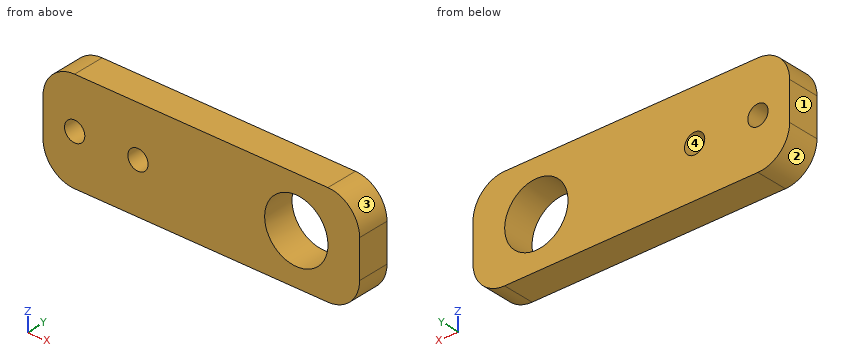
from build123d import *

# Parameters (mm, degrees)
SKETCH1_W           = 50
SKETCH1_H           = 16
SKETCH1_R           = 5
SKETCH1_R_2         = 1.6
BOSS_EXTRUDE1_DEPTH = 5
FILLET1_R           = 5


with BuildPart() as part:
    # Sketch1 → Boss-Extrude1 (new body)
    with BuildSketch(Plane(origin=(0, 0, 0), x_dir=(1, 0, 0), z_dir=(0, 1, 0))):
        with Locations((25, 8)):
            Rectangle(SKETCH1_W, SKETCH1_H)
        with Locations(Location((40, 8, 0), (0, 0, 270))):
            Circle(SKETCH1_R, mode=Mode.SUBTRACT)
        with Locations(Location((5, 8, 0), (0, 0, 270))):
            Circle(SKETCH1_R_2, mode=Mode.SUBTRACT)
        with Locations(Location((15, 8, 0), (0, 0, 270))):
            Circle(SKETCH1_R_2, mode=Mode.SUBTRACT)
    extrude(amount=BOSS_EXTRUDE1_DEPTH)

    # Fillet1
    fillet1_edges = [part.edges().sort_by_distance(p)[0] for p in [
        (0, 2.5, -16),
        (50, 2.5, -16),
        (50, 2.5, 0),
        (0, 2.5, 0),
    ]]
    fillet(fillet1_edges, radius=FILLET1_R)


solid = part.part
The listing builds one solid part. Answer for the finished solid, in the listing's coordinates (mm). Face numbers are marked on the shaded views. Give positions to 0.01 mm unless a question says otherwise; leave off trailing zeros. Write each loop counter-clockwise with the first axis right and the second up, starting at its lowest first coordinate (ties: lowest second). Pieces come first, ordered by that corner, then holes.
Item 1: Find the intervals of material crossed by line 1 along X through (y, z) = (3.9, -8); line 2 along X through (y, z) = (0.9, -7); line 3 along Z through (x, y) = (37.5, 3.9), in increasing order.
Item 2: Section D-D, the plane x = 40 is taken. Write down the section's boundary in (y, z), plus the area to 3 significant figures.
Item 3: Flat-ended cylindrical pins translate along their axes: P1, Ø3, axis at y = 1.5, z = -2, coming from the +X side; P2, Ø1.9, axis at x = 15, z = -8, coming from the -Y side; P3, Ø1, axis at y = 3.5, z = -3, coming from the -X side. Find the tip coordinate at first contact, or state that the pin passes through.
Item 4: Determine the mould class of the marked faces 1, 2, 3 and 4 for opening direction Z: released by +Z, released by -Z, zero draft, split by the parting line, or undercut.
Item 5: Section C-C, the plane y = 3.45 is taken. Write down the section's boundary in (x, z).
Item 6: Section A-A, the plane z = -8 is taken. Write down the section's boundary in (x, y), plus the area to 3 significant figures.
Item 7: Section B-B, the plane x = 15 is taken. Write down the section's boundary in (y, z).
Completed:
1. line 1: x = 0 to 3.4, 6.6 to 13.4, 16.6 to 35, 45 to 50
1. line 2: x = 0 to 3.75, 6.25 to 13.75, 16.25 to 35.1, 44.9 to 50
1. line 3: z = -16 to -12.33, -3.67 to 0
2. outline: (0, -16) - (5, -16) - (5, -13) - (0, -13) - close; (0, -3) - (5, -3) - (5, 0) - (0, 0) - close
2. area: 30.0 mm2
3. P1: stops at x = 49.77
3. P2: passes through
3. P3: stops at x = 0.23
4. face 1: zero draft
4. face 2: released by -Z
4. face 3: released by +Z
4. face 4: undercut
5. outline: (0, -11) arc R5 ccw to (5, -16) - (45, -16) arc R5 ccw to (50, -11) - (50, -5) arc R5 ccw to (45, 0) - (5, 0) arc R5 ccw to (0, -5) - close; hole circle Ø3.2 at (5, -8); hole circle Ø3.2 at (15, -8); hole circle Ø10 at (40, -8)
6. outline: (0, 0) - (3.4, 0) - (3.4, 5) - (0, 5) - close; (6.6, 0) - (13.4, 0) - (13.4, 5) - (6.6, 5) - close; (16.6, 0) - (35, 0) - (35, 5) - (16.6, 5) - close; (45, 0) - (50, 0) - (50, 5) - (45, 5) - close
6. area: 168 mm2
7. outline: (0, -16) - (5, -16) - (5, -9.6) - (0, -9.6) - close; (0, -6.4) - (5, -6.4) - (5, 0) - (0, 0) - close
